Input: dimensioned drawing with shaded views. Units: mm. Origin: part minimum x, y, z. A direction names the side the tool comes from. Give positions to 0.01 mm unless a question says otherwise; leave off trailing zeros. Write each loop counter-clockwise with the first axis right and the second up, starting at its lowest first coordinate (ties: lowest second). Pieces come first, ordered by that corner, then holes. Notation, with made-up numbers: (1.25, -11) -> (38.25, -11) arc R7 ccw to (38.25, -3) -> close; hole circle Ø5 at (-26.5, 18). An arc over 180 degrees is marked (long way). Answer as a JSON object with one key per item and string values. Group by question number.
(1) Draft query along X for the marked faces 1, 2 and 3. Return one class per face: +X half, -X half, draft (parallel to the pull), parting line (faces both ways), or undercut.
(2) Section query B-B on x = 19.75. Output: boundary loops of the cut face in (y, z).
(3) Contact query for flat-ended pins moving along their axis: pin 1 Ø4 at (x, y) = (17.5, 14) entering from +Z; pin 2 Ø4 at (y, z) = (10, 33.5) entering from -X; pin 3 Ø1.5 at (x, y) = (20, 13) entering from -Z. Output: stop coordinate, or through.
(4) Material intervals for probe 1 along X at (y, z) = (10, 7.9); probe 2 along Y at (x, z) = (1.4, 18); probe 3 along Z at (x, y) = (6.5, 1.5), sorted ascending.
(5) Section query C-C on x = 23. Output: boundary loops of the cut face in (y, z).
(6) Section query D-D on y = 10. Output: boundary loops of the cut face in (x, z).
(7) Set-up query: the marked faces 4, 5 and 6. Return all of +Z, -Z, +X, -X, +Y, -Y with unobstructed straight access to the full face (end or side cutting, diameter ignored); none if empty.
(8) Section query A-A on z = 18. Output: boundary loops of the cut face in (x, y).
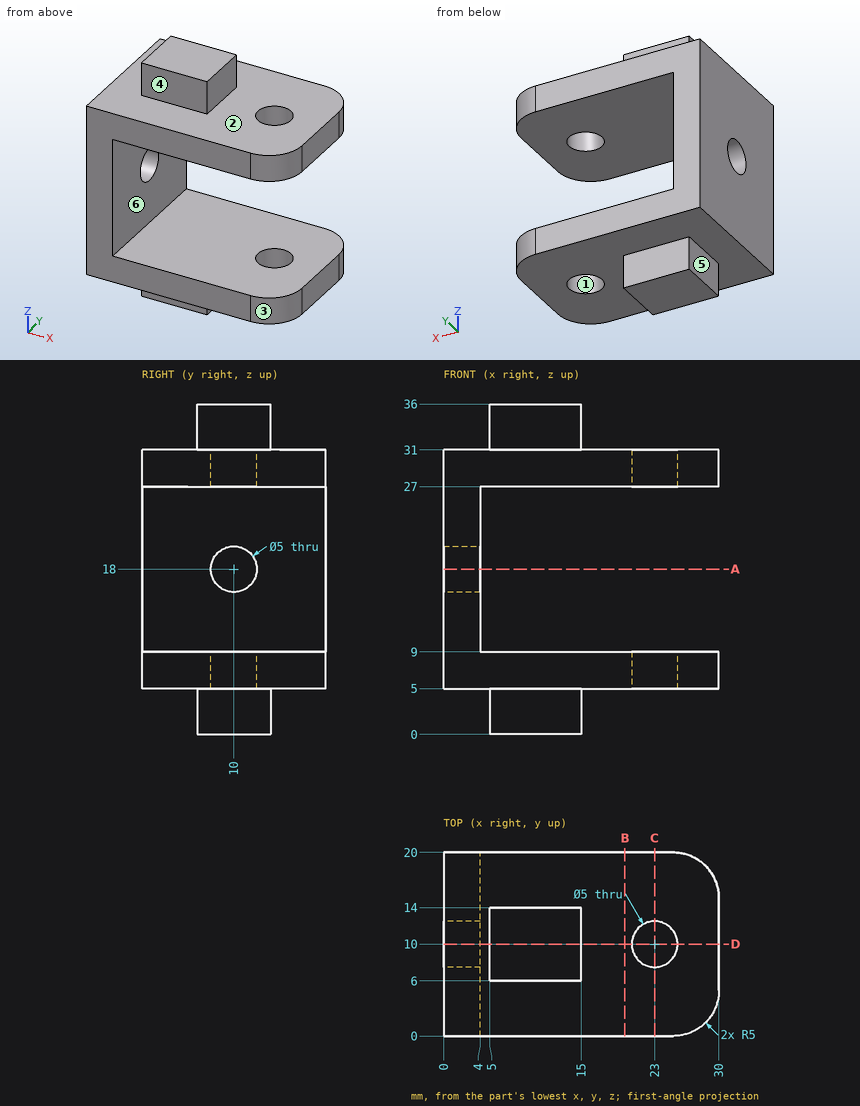
Answer list:
{
 "1": {"face 1": "undercut", "face 2": "draft", "face 3": "+X half"},
 "2": {"outline": "(0, 5) -> (20, 5) -> (20, 9) -> (0, 9) -> close; (0, 27) -> (20, 27) -> (20, 31) -> (0, 31) -> close"},
 "3": {"pin 1": "z = 31", "pin 2": "x = 5", "pin 3": "z = 5"},
 "4": {"probe 1": "0 to 20.5, 25.5 to 30", "probe 2": "0 to 7.5, 12.5 to 20", "probe 3": "5 to 9, 27 to 31"},
 "5": {"outline": "(0, 5) -> (7.5, 5) -> (7.5, 9) -> (0, 9) -> close; (0, 27) -> (7.5, 27) -> (7.5, 31) -> (0, 31) -> close; (12.5, 5) -> (20, 5) -> (20, 9) -> (12.5, 9) -> close; (12.5, 27) -> (20, 27) -> (20, 31) -> (12.5, 31) -> close"},
 "6": {"outline": "(0, 5) -> (5, 5) -> (5, 0) -> (15, 0) -> (15, 5) -> (20.5, 5) -> (20.5, 9) -> (4, 9) -> (4, 15.5) -> (0, 15.5) -> close; (0, 20.5) -> (4, 20.5) -> (4, 27) -> (20.5, 27) -> (20.5, 31) -> (15, 31) -> (15, 36) -> (5, 36) -> (5, 31) -> (0, 31) -> close; (25.5, 5) -> (30, 5) -> (30, 9) -> (25.5, 9) -> close; (25.5, 27) -> (30, 27) -> (30, 31) -> (25.5, 31) -> close"},
 "7": {"face 4": "+Z, +X, -X, -Y", "face 5": "-Z, -X, +Y, -Y", "face 6": "+X, +Y, -Y"},
 "8": {"outline": "(0, 0) -> (4, 0) -> (4, 7.5) -> (0, 7.5) -> close; (0, 12.5) -> (4, 12.5) -> (4, 20) -> (0, 20) -> close"}
}
